Design review of the part built by this model. Coordinates are the model's own, in mm. Face numbers are marked on the shaded views. A direction names the side the tool comes from. Coordinates: 2 decimals unless noted, no trailing zeros. Loops run counter-clockwise (first coordinate to the right, second up) from the corner with the lowest first, then second, coordinate; pieces in that order, holes last. Notation, with made-up numbers: M 84.5,71.5 L 113.5,71.5 A10 cw 113.5,75.5 Z; hole C -27,75 d9. An arc over 180 degrees is marked long. Write item = value, one per line. Start each with the question number.
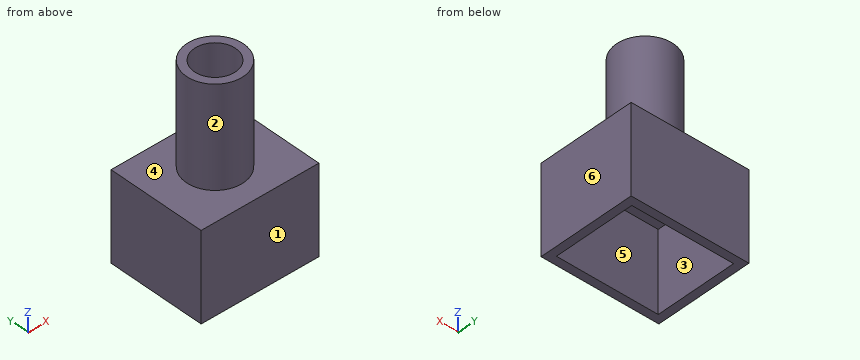
from build123d import *

# Parameters (mm, degrees)
F0_W      = 29.5
F0_H      = 24.5
F0_W_2    = 25.5
F0_H_2    = 20.5
F1_DEPTH  = 20
F2_W      = 29.5
F2_H      = 24.5
F3_DEPTH  = 2
F4_R      = 7.15
F4_R_2    = 5.15
F5_DEPTH  = 25
F5_FACE_R = 5.15
F6_DEPTH  = 25


with BuildPart() as f1:
    # F0 (on Top) → F1 (new body)
    with BuildSketch(Plane.XY):
        Rectangle(F0_W, F0_H)
        Rectangle(F0_W_2, F0_H_2, mode=Mode.SUBTRACT)
    extrude(amount=F1_DEPTH)

    # F2 (on face) → F3 (join)
    with BuildSketch(Plane.XY.offset(20)):
        Rectangle(F2_W, F2_H)
    extrude(amount=F3_DEPTH)

    # F4 (on face) → F5 (join)
    with BuildSketch(Plane.XY.offset(22)):
        Circle(F4_R)
        Circle(F4_R_2, mode=Mode.SUBTRACT)
    extrude(amount=F5_DEPTH)

    # F5_face (on face) → F6 (cut)
    with BuildSketch(Plane.XY.offset(22)):
        Circle(F5_FACE_R)
    extrude(amount=-F6_DEPTH, mode=Mode.SUBTRACT)


solid = f1.part
Q1. Add section D-D on z = 29. State the section outline as (x, y) points.
Q2. Clearance check with flat-ended pins moving along their axes: P1, Ø8, axis at x = 0, y = 0, coming from the +Z side; P2, Ø2, axis at x = 0.5, z = 27, coming from the +Y side; P3, Ø4, axis at x = -2.5, z = 28, coming from the -Y side; P4, Ø3, axis at x = -1, y = 7, coming from the -Z side. State where each tip first meets the part, or that it passes through.
Q3. Mouldability with a two-part tool opening along Y and no side actions: class the marked faces 1, 2 and 3 as released by +Y, released by -Y, zero draft, split by the parting line, or undercut.
Q4. For the marked faces 4, 5 and 6, list the 3-axis set-ups (+Z, -Z, +X, -X, +Y, -Y) from which the entire face can be reached by the end or side of a thin tool; tool diameter is ignored.
Q5. Add section A-A on y = 0. State the section outline as (x, z) points.
Q6. Add section B-B on x = 0. State the section outline as (y, z) points.
Q7. Add section C-C on x = -11. State the section outline as (y, z) points, plus the area to 3 significant figures.
Q8. To check wall thickness, follow line 1 (Y direction, x = 0, z = 21); line 2 (Y direction, x = 4.75, z = 19); line 3 (X direction, y = -2.25, z = 18). State the ranges of each line that lie inside material, in increasing order. Write a range as from..to.
Values follow:
q1.outline = C 0,0 d14.3; hole C 0,0 d10.3
q2.P1 = through
q2.P2 = 7.15
q2.P3 = -7.13
q2.P4 = 20
q3.face_1 = released by -Y
q3.face_2 = split by the parting line
q3.face_3 = undercut
q4.face_4 = +Z
q4.face_5 = -Z
q4.face_6 = +Z, -Z, +X, +Y, -Y
q5.outline = M -14.75,0 L -12.75,0 L -12.75,20 L -5.15,20 L -5.15,47 L -7.15,47 L -7.15,22 L -14.75,22 Z; M 5.15,20 L 12.75,20 L 12.75,0 L 14.75,0 L 14.75,22 L 7.15,22 L 7.15,47 L 5.15,47 Z
q6.outline = M -12.25,0 L -10.25,0 L -10.25,20 L -5.15,20 L -5.15,47 L -7.15,47 L -7.15,22 L -12.25,22 Z; M 5.15,20 L 10.25,20 L 10.25,0 L 12.25,0 L 12.25,22 L 7.15,22 L 7.15,47 L 5.15,47 Z
q7.outline = M -12.25,0 L -10.25,0 L -10.25,20 L 10.25,20 L 10.25,0 L 12.25,0 L 12.25,22 L -12.25,22 Z
q7.area = 129 mm2
q8.line_1 = -12.25..-5.15, 5.15..12.25
q8.line_2 = -12.25..-10.25, 10.25..12.25
q8.line_3 = -14.75..-12.75, 12.75..14.75
